```python
from build123d import *

# Parameters (mm, degrees)
F0_W     = 50
F0_H     = 50
F1_DEPTH = 48
F2_T     = -2
F3_W     = 10
F3_H     = 10
F5_DEPTH = 2
F4_W     = 10
F4_H     = 10
F6_DEPTH = 2


with BuildPart() as f1:
    # F0 (on Top) → F1 (new body)
    with BuildSketch(Plane.XY):
        with Locations((-1.763418, 5.553549)):
            Rectangle(F0_W, F0_H)
    extrude(amount=F1_DEPTH)

    # F2
    f2_openings = [f1.faces().sort_by_distance(p)[0] for p in [
        (-1.763418, 5.553549, 48),
    ]]
    offset(amount=F2_T, openings=f2_openings)

    # F3 (on face) → F5 (cut)
    with BuildSketch(Plane.XZ.offset(19.446451)):
        with Locations((-16.763418, 38)):
            Rectangle(F3_W, F3_H)
        with Locations((13.236582, 10)):
            Rectangle(F3_W, F3_H)
    extrude(amount=-F5_DEPTH, mode=Mode.SUBTRACT)

    # F4 (on face) → F6 (cut)
    with BuildSketch(Plane(origin=(0, 30.553549, 0), x_dir=(-1, 0, 0), z_dir=(0, 1, 0))):
        with Locations((16.763418, 38)):
            Rectangle(F4_W, F4_H)
        with Locations((-13.236582, 10)):
            Rectangle(F4_W, F4_H)
    extrude(amount=-F6_DEPTH, mode=Mode.SUBTRACT)


solid = f1.part
```
For this review, take the finished solid that the model builds, in its own axes (mm). A direction names the side the tool comes from. Coordinates: 2 decimals unless noted, no trailing zeros. Write each loop counter-clockwise with the first axis right and the second up, starting at its lowest first coordinate (ties: lowest second). Pieces come first, ordered by that corner, then holes. Notation, with made-up numbers: (67.25, 0) - (121.25, 0) arc R25 cw to (121.25, 19) - close; hole circle Ø2 at (-28.75, 62.25). An arc over 180 degrees is marked (long way). Answer in a Markdown table with one row per item. Add a question column.
Q1. For P1, Ø5, axis at x = 6, y = 9.5, coming from the +Z side, flat-tipped, find the tip position at first contact; note if it passes through.
Q2. We need section B-B, the plane z = 11. State the section outline as (x, y) points, and give its area (3 significant figures).
Q3. We need section A-A, the plane x = -15.5. State the section outline as (y, z) points, and give its area (3 significant figures).
Q4. We need section D-D, the plane y = 13. State the section outline as (x, z) points, and give its area (3 significant figures).
Q5. For probe 1 along Y at (x, z) = (-7, 31.5); probe 2 along X at (y, z) = (3.5, 24); probe 3 along Z at (x, y) = (-6, 28.5), list the stretches that pass through material, from the lowest coordinate up.
Q6. We need section C-C, the plane z = 22.5. State the section outline as (x, y) points, and give its area (3 significant figures).
Q7. Draft analysis for pull direction Z (two halves, no side actions). For faces 1 (the flat face through (21.237, 5, 25)), 2 (the flat face through (18.237, 30, 10)), 3 (the flat face through (-2, 6, 0)), state which applies: +Z half, -Z half, draft (parallel to the pull), parting line (faces both ways), or undercut.
Q8. Tool access review of faces 4 (the flat face through (-2, 28.554, 25)), 5 (the flat face through (-17, 30, 33)), 6 (the flat face through (23.237, 5, 24)): name each direction out of +Z, -Z, +X, -X, +Y, -Y from which nothing blocks a thin tool from reaching the whole face with its end or side.
Answer list:
| question | item | result |
|---|---|---|
| 1 | P1 | stops at z = 2 |
| 2 | outline | (-26.76, -19.45) - (8.24, -19.45) - (8.24, -17.45) - (-24.76, -17.45) - (-24.76, 28.55) - (8.24, 28.55) - (8.24, 30.55) - (-26.76, 30.55) - close; (18.24, -19.45) - (23.24, -19.45) - (23.24, 30.55) - (18.24, 30.55) - (18.24, 28.55) - (21.24, 28.55) - (21.24, -17.45) - (18.24, -17.45) - close |
| 2 | area | 344 mm2 |
| 3 | outline | (-19.45, 0) - (30.55, 0) - (30.55, 33) - (28.55, 33) - (28.55, 2) - (-17.45, 2) - (-17.45, 33) - (-19.45, 33) - close; (-19.45, 43) - (-17.45, 43) - (-17.45, 48) - (-19.45, 48) - close; (28.55, 43) - (30.55, 43) - (30.55, 48) - (28.55, 48) - close |
| 3 | area | 244 mm2 |
| 4 | outline | (-26.76, 0) - (23.24, 0) - (23.24, 48) - (21.24, 48) - (21.24, 2) - (-24.76, 2) - (-24.76, 48) - (-26.76, 48) - close |
| 4 | area | 284 mm2 |
| 5 | probe 1 | y = -19.45 to -17.45, 28.55 to 30.55 |
| 5 | probe 2 | x = -26.76 to -24.76, 21.24 to 23.24 |
| 5 | probe 3 | z = 0 to 2 |
| 6 | outline | (-26.76, -19.45) - (23.24, -19.45) - (23.24, 30.55) - (-26.76, 30.55) - close; hole (-24.76, -17.45) - (21.24, -17.45) - (21.24, 28.55) - (-24.76, 28.55) - close |
| 6 | area | 384 mm2 |
| 7 | face 1 | draft |
| 7 | face 2 | undercut |
| 7 | face 3 | -Z half |
| 8 | face 4 | +Z |
| 8 | face 5 | +Y, -Y |
| 8 | face 6 | +Z, -Z, +X, +Y, -Y |
